Model file for the job. Use its own axes, mm. A direction names the side the tool comes from. Give positions to 0.01 mm unless a question says otherwise; leave off trailing zeros. Loops run counter-clockwise (first coordinate to the right, second up) from the corner with the lowest first, then second, coordinate; pieces in that order, holes last. Notation, with made-up numbers: (-17.5, 35) -> (10.5, 35) arc R32 ccw to (10.5, 70) -> close; hole circle Ø11 at (29.25, -11.75). An arc over 180 degrees is marked (long way). Use CSV: the item, a comma, the result in double quotes. Start each with the question number.
(1) Cut at B-B on x = -48.5. Write the cut outline in (y, z).
(2) Flat gauge pins, fed straight in: pin 1 (1.6 mm diameter, centred on y = 1, z = 22.5, fed in from +X); pin 2 (12 mm diameter, centred on x = -30, z = 39, fed in from -Y); pin 3 (3.5 mm diameter, centred on x = 4.5, y = 15, fed in from -Z). Where does each tip first touch, or does it go through?
(3) Cut at D-D on x = -27. Write the cut outline in (y, z).
(4) 3-axis set-ups, long thin cutter, end or side, ignore diameter. For faces 1 (the flat face through (-49, 2, 16)), 2 (the flat face through (-20.6, 27, 16)), 3 (the cylindrical face through (-9, 19, 16)), 4 (the flat face through (-21, 21, 37)), 5 (the flat face through (-54, 1, 16)): which of +Z, -Z, +X, -X, +Y, -Y reach the whole face in a straight line?
(5) Cut at C-C on y = 5. Write the cut outline in (x, z), then the cut area to 3 significant figures.
(6) Drill centre lines: probe 1 along X at (y, z) = (41.55, 16); probe 2 along Z at (x, y) = (-27, 42.05); probe 3 along Y at (x, z) = (-8, 16). Where is each one in solid material? Low to high.
(7) Pull direction Y, two halves, no side cores. Call faces 6 (the flat face through (4, 26, 4)), 7 (the flat face through (-27, 21, 0)), 8 (the flat face through (-27, 13, 16)), 9 (the flat face through (2.75, 24, 16)): pulls with the +Y half, pulls with the -Y half, needs draft (parallel to the pull), parting line crosses it, or undercut.
(8) Cut at A-A on y = 28.5. Write the cut outline in (x, z), then the cut area to 3 significant figures.
Autodesk Inventor part; units mm, degrees
ref_plane "YZ Plane" through (0, 0, 0) normal (1, 0, 0) x (0, 1, 0)
ref_plane "XZ Plane" through (0, 0, 0) normal (0, 1, 0) x (-1, 0, 0)
ref_plane "XY Plane" through (0, 0, 0) normal (0, 0, 1) x (1, 0, 0)
sketch "Sketch1" plane through (0, 0, 0) normal (1, 0, 0) x (0, 1, 0)
  point P0 (0, 0)
sketch "Sketch2" plane through (0, 0, 0) normal (1, 0, 0) x (0, 1, 0)
  point P0 (0, 0)
sketch "Sketch3" plane through (0, 0, 0) normal (0, 1, 0) x (-1, 0, 0)
  point P0 (0, 0)
sketch "Sketch4" plane through (0, 0, 0) normal (0, 1, 0) x (-1, 0, 0)
  line L0 (52, 32) -> (2, 32)
  line L1 (0, 30) -> (0, 2)
  line L2 (2, 0) -> (52, 0)
  line L3 (54, 2) -> (54, 30)
  arc A0 (2, 32) -> (0, 30) centre (2, 30) ccw
  arc A1 (0, 2) -> (2, 0) centre (2, 2) ccw
  arc A2 (52, 0) -> (54, 2) centre (52, 2) ccw
  arc A3 (54, 30) -> (52, 32) centre (52, 30) ccw
  point P0 (0, 0)
  dimension "d0" = 2
extrude "Extrusion1" add sketch "Sketch4" along normal blind 2
sketch "Sketch5" plane through (0, 2, 0) normal (0, 1, 0) x (1, 0, 0)
  point P0 (0, 0)
sketch "Sketch6" plane through (0, 2, 0) normal (0, 1, 0) x (1, 0, 0)
  point P0 (0, 0)
sketch "Sketch7" plane through (0, 2, 0) normal (0, 1, 0) x (1, 0, 0)
  line L0 (-11, 0) -> (-43, 0)
  line L1 (-43, 0) -> (-43, -32)
  line L2 (-43, -32) -> (-11, -32)
  line L3 (-11, -32) -> (-11, 0)
  point P0 (0, 0)
extrude "Extrusion2" add sketch "Sketch7" along normal blind 41
fillet "Fillet1" radius 1 1 edges at (-11, 2, 16)
fillet "Fillet2" radius 1 1 edges at (-43, 2, 16)
sketch "Sketch8" plane through (-52, 0, 32) normal (0, 0, 1) x (1, 0, 0)
  point P0 (52, 0)
sketch "Sketch9" plane through (-52, 0, 32) normal (0, 0, 1) x (1, 0, 0)
  line L0 (19, 15.5) -> (31, 15.5)
  line L1 (31, 15.5) -> (31, 27.5)
  line L2 (31, 27.5) -> (19, 27.5)
  line L3 (19, 27.5) -> (19, 15.5)
  point P0 (52, 0)
sketch "Sketch10" plane through (-11, 43, 32) normal (1, 0, 0) x (0, 0, -1)
  line L0 (10, -15.5) -> (22, -15.5)
  line L1 (22, -15.5) -> (22, -27.5)
  line L2 (22, -27.5) -> (10, -27.5)
  line L3 (10, -27.5) -> (10, -15.5)
  point P0 (32, -43)
sketch "Sketch11" plane through (0, 43, 0) normal (0, 1, 0) x (1, 0, 0)
  line L0 (-43, -32) -> (-43, 0)
  line L1 (-11, 0) -> (-43, 0)
  line L2 (-2, 0) -> (-52, 0)
  circle A0 centre (-27, -16) radius 9.5
  point P0 (0, 0)
sketch "Sketch12" plane through (0, 43, 0) normal (0, 1, 0) x (1, 0, 0)
  point P0 (0, 0)
sketch "Sketch13" plane through (0, 43, 0) normal (0, 1, 0) x (1, 0, 0)
  point P0 (0, 0)
extrude "Extrusion3" cut sketch "Sketch11" along normal blind 2
sketch "Sketch14" plane through (0, 43, 0) normal (0, 1, 0) x (1, 0, 0)
  line L0 (-43, 0) -> (-43, -32)
  line L1 (-11, -32) -> (-11, 0)
  line L2 (-10, -32) -> (-10, 0)
  point P0 (0, 0)
sketch "Sketch15" plane through (0, 43, 0) normal (0, 1, 0) x (1, 0, 0)
  line L0 (-20.6, -9.6) -> (-33.4, -9.6)
  line L1 (-33.4, -9.6) -> (-33.4, -22.4)
  line L2 (-33.4, -22.4) -> (-20.6, -22.4)
  line L3 (-20.6, -22.4) -> (-20.6, -9.6)
  point P0 (0, 0)
sketch "Sketch16" plane through (0, 43, 0) normal (0, 1, 0) x (1, 0, 0)
  point P0 (0, 0)
sketch "Sketch17" plane through (0, 43, 0) normal (0, 1, 0) x (1, 0, 0)
  point P0 (0, 0)
extrude "Extrusion4" cut sketch "Sketch15" against normal blind 30
sketch "Sketch18" plane through (0, 43, 0) normal (0, 1, 0) x (1, 0, 0)
  point P0 (0, 0)
sketch "Sketch19" plane through (0, 43, 0) normal (0, 1, 0) x (1, 0, 0)
  circle A0 centre (-27, -16) radius 9.5
  point P0 (0, 0)
extrude "Extrusion5" cut sketch "Sketch19" against normal blind 2
sketch "Sketch20" plane through (-43, 43, 0) normal (-1, 0, 0) x (0, 0, 1)
  line L0 (10, -10) -> (22, -10)
  line L1 (22, -10) -> (22, -31)
  line L2 (22, -31) -> (10, -31)
  line L3 (10, -31) -> (10, -10)
  point P0 (0, -43)
extrude "Extrusion6" add sketch "Sketch10" along normal blind 11
extrude "Extrusion7" add sketch "Sketch9" along normal blind 11
extrude "Extrusion8" add sketch "Sketch20" along normal blind 11
sketch "Sketch21" plane through (0, 43, 32) normal (1, 0, 0) x (0, 0, -1)
  line L0 (2.5, -12) -> (29.5, -12)
  line L1 (29.5, -12) -> (29.5, -31)
  line L2 (29.5, -31) -> (2.5, -31)
  line L3 (2.5, -31) -> (2.5, -12)
  point P0 (32, -43)
sketch "Sketch22" plane through (-52, 0, 43) normal (0, 0, 1) x (1, 0, 0)
  line L0 (15.5, 2.5) -> (34.5, 2.5)
  line L1 (34.5, 2.5) -> (34.5, 42.5)
  line L2 (34.5, 42.5) -> (15.5, 42.5)
  line L3 (15.5, 42.5) -> (15.5, 2.5)
  point P0 (52, 0)
extrude "Extrusion9" add sketch "Sketch21" along normal blind 6
extrude "Extrusion10" add sketch "Sketch22" along normal blind 6
sketch "Sketch23" plane through (-54, 43, 0) normal (-1, 0, 0) x (0, 0, 1)
  line L0 (3.5, -40) -> (28.5, -40)
  line L1 (28.5, -40) -> (28.5, 12)
  line L2 (28.5, 12) -> (3.5, 12)
  line L3 (3.5, 12) -> (3.5, -40)
  point P0 (0, -43)
extrude "Extrusion11" add sketch "Sketch23" along normal blind 2
sketch "Sketch24" plane through (6, 43, 32) normal (1, 0, 0) x (0, 0, -1)
  line L0 (16, -22) -> (-30.5795, -61.0635)
  point P0 (32, -43)
hole "Hole1" at (6, 21, 16) direction (-1, 0, 0) diameter 4 depth 27 tip angle 118
sketch "Sketch25" plane through (6, 43, 32) normal (1, 0, 0) x (0, 0, -1)
  line L0 (7.5, -17) -> (7.5, -13)
  line L1 (29.5, -12) -> (2.5, -12)
  line L2 (7.5, -13) -> (24.5, -13)
  line L3 (24.5, -13) -> (24.5, -16.5)
  line L4 (24.5, -16.5) -> (26.5, -16.5)
  line L5 (26.5, -16.5) -> (26.5, -17)
  line L6 (26.5, -17) -> (28.5, -17)
  line L7 (28.5, -26) -> (24.5, -26)
  line L8 (24.5, -26) -> (24.5, -30)
  line L9 (24.5, -30) -> (7.5, -30)
  line L10 (22.4, -30) -> (9.6, -30)
  line L11 (7.5, -30) -> (7.5, -26)
  line L12 (7.5, -26) -> (3.5, -26)
  line L13 (3.5, -17) -> (7.5, -17)
  line L14 (28.5, -17) -> (29.5, -17)
  line L15 (29.5, -31) -> (29.5, -12)
  line L16 (28.5, -26) -> (29.5, -26)
  line L17 (29.5, -26) -> (29.5, -17)
  line L18 (3.5, -17) -> (2.5, -17)
  line L19 (2.5, -17) -> (2.5, -26)
  line L20 (2.5, -26) -> (3.5, -26)
  point P0 (32, -43)
extrude "Extrusion12" cut sketch "Sketch25" against normal blind 3.25
properties part number "Cuvette Holder"
Check result:
1,outline,"(0, 0) -> (2, 0) -> (2, 32) -> (0, 32) -> close; (12, 10) -> (33, 10) -> (33, 22) -> (12, 22) -> close"
2,pin 1,"x = 0"
2,pin 2,"y = 2.5"
2,pin 3,"z = 2.5"
3,outline,"(0, 0) -> (43, 0) -> (43, 6.5) -> (41, 6.5) -> (41, 9.6) -> (13, 9.6) -> (13, 22.4) -> (41, 22.4) -> (41, 25.5) -> (43, 25.5) -> (43, 32) -> (27.5, 32) -> (27.5, 43) -> (42.5, 43) -> (42.5, 49) -> (2.5, 49) -> (2.5, 43) -> (15.5, 43) -> (15.5, 32) -> (0, 32) -> close"
4,face 1,"+Z, -Z, -X"
4,face 2,"+Y"
4,face 3,"+X"
4,face 4,"+X, +Y, -Y"
4,face 5,"+Z, -Z, -X, -Y"
5,outline,"(-56, 3.5) -> (-54, 3.5) -> (-54, 28.5) -> (-56, 28.5) -> close; (-43, 0) -> (-11, 0) -> (-11, 32) -> (-43, 32) -> close; (-36.5, 43) -> (-17.5, 43) -> (-17.5, 49) -> (-36.5, 49) -> close"
5,area,"1,190 mm²"
6,probe 1,"-56 to -54, -43 to -36.5, -17.5 to -11"
6,probe 2,"0 to 6.5, 25.5 to 32, 43 to 49"
6,probe 3,"0 to 2, 15.5 to 19, 23 to 27.5"
7,face 6,"undercut"
7,face 7,"needs draft"
7,face 8,"pulls with the +Y half"
7,face 9,"undercut"
8,outline,"(-56, 3.5) -> (-54, 3.5) -> (-54, 10) -> (-43, 10) -> (-43, 0) -> (-11, 0) -> (-11, 32) -> (-43, 32) -> (-43, 22) -> (-54, 22) -> (-54, 28.5) -> (-56, 28.5) -> close; (-36.5, 43) -> (-17.5, 43) -> (-17.5, 49) -> (-36.5, 49) -> close; (0, 2.5) -> (6, 2.5) -> (6, 7.5) -> (2.75, 7.5) -> (2.75, 24.5) -> (6, 24.5) -> (6, 29.5) -> (0, 29.5) -> close; hole (-33.4, 9.6) -> (-20.6, 9.6) -> (-20.6, 22.4) -> (-33.4, 22.4) -> close"
8,area,"1,260 mm²"
